Drawing for the job (mm, zero at the part's lowest x, y, z). A direction names the side the tool comes from. Round coordinates to 2 decimals unless told otherwise and drop trailing zeros. Write each loop counter-clockwise with the first axis right and the second up, starting at its lowest first coordinate (ties: lowest second). Pieces come first, ordered by that corner, then holes. Notation, with made-up numbers: M 49,-13.75 L 107,-13.75 A25 ccw 107,24.25 Z; hole C 89.25,17.25 d9. An arc over 180 degrees is marked long. Use a Markdown table: item, result. Add a question column.
1) Wall check: probe 1 along Y at (x, z) = (17.75, 13) (1 decimal); probe 2 along X at (y, z) = (19, 9.5); probe 3 along Y at (x, z) = (6, 3.5) (1 decimal). Give the ranges that are in metal, low to high.
2) Slice it at C-C on y = 56.5. Write the cut outline in (x, z) (1 decimal).
3) Two-plate mould, pull along X, no slides. Class the marked faces 3, 4 and 5: released by +X, released by -X, zero draft, split by the parting line, or undercut.
4) Slice it at A-A on z = 7.75. Write the cut outline in (x, y) (1 decimal).
5) Slice it at B-B on x = 18.5. Write the cut outline in (y, z) (1 decimal).
6) Which spindle directions (+Z, -Z, +X, -X, +Y, -Y) get a long thin tool onto all of the face, cutting with end or side? Do the marked faces 1 and 2. Say none if no direction does.
7) Drop flat-ended pins along their axis: P1, Ø10, axis at y = 58, z = 7.5, coming from the -X side; P2, Ø1.5, axis at x = 13.5, y = 40.5, coming from the -Z side; P3, Ø1, axis at x = 4.5, z = 8.5, coming from the -Y side (1 decimal); P4, Ø4, axis at x = 19.5, z = 10.5, coming from the -Y side. Give the stop position or say it passes through.
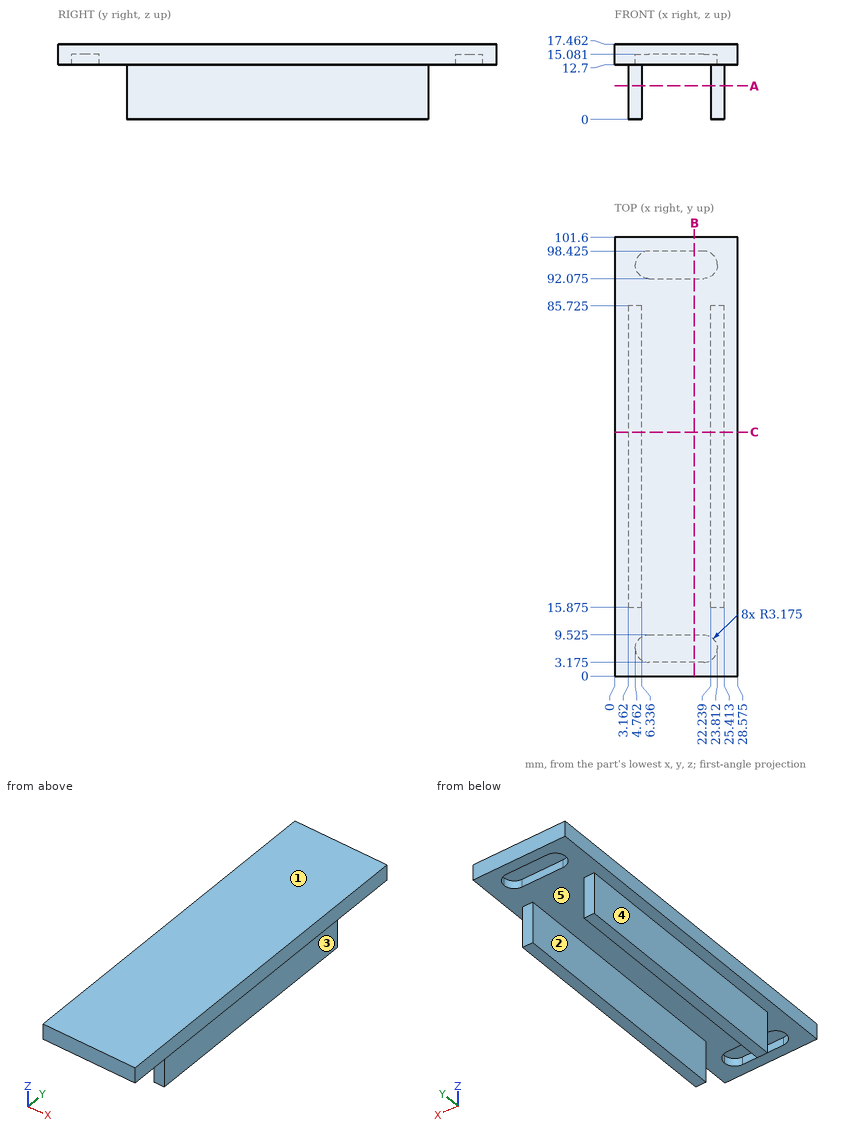
Entries:
| question | item | result |
|---|---|---|
| 1 | probe 1 | y = 0 to 3.2, 9.5 to 92.1, 98.4 to 101.6 |
| 1 | probe 2 | x = 3.16 to 6.34, 22.24 to 25.41 |
| 1 | probe 3 | y = 15.9 to 85.7 |
| 2 | outline | M 0,12.7 L 3.2,12.7 L 3.2,0 L 6.3,0 L 6.3,12.7 L 22.2,12.7 L 22.2,0 L 25.4,0 L 25.4,12.7 L 28.6,12.7 L 28.6,17.5 L 0,17.5 Z |
| 3 | face 3 | released by +X |
| 3 | face 4 | released by -X |
| 3 | face 5 | undercut |
| 4 | outline | M 3.2,15.9 L 6.3,15.9 L 6.3,85.7 L 3.2,85.7 Z; M 22.2,15.9 L 25.4,15.9 L 25.4,85.7 L 22.2,85.7 Z |
| 5 | outline | M 0,12.7 L 3.2,12.7 L 3.2,15.1 L 9.5,15.1 L 9.5,12.7 L 92.1,12.7 L 92.1,15.1 L 98.4,15.1 L 98.4,12.7 L 101.6,12.7 L 101.6,17.5 L 0,17.5 Z |
| 6 | face 1 | +Z, +X, -X, +Y, -Y |
| 6 | face 2 | -Z, +Y, -Y |
| 7 | P1 | stops at x = 3.16 |
| 7 | P2 | stops at z = 12.7 |
| 7 | P3 | stops at y = 15.9 |
| 7 | P4 | passes through |
